Build history of the part. All positions in model axes, mm. A direction names the side the tool comes from. Give positions to 0.01 mm unless a question says otherwise; leave off trailing zeros. Loops run counter-clockwise (first coordinate to the right, second up) from the corner with the lowest first, then second, coordinate; pieces in that order, holes last.
1) Wall check: line 1 (X direction, y = -24.5, z = 0); line 2 (Z direction, x = 1, y = 50); line 3 (Z direction, x = -3.5, y = -19.5). Give the ranges that are in metal, low to high.
2) Band-saw the part on C-C on y = -2.5. List the corners of the cut face in (x, z).
3) Band-saw the part on A-A on y = -21.5. List the corners of the cut face in (x, z), then the cut area to 3 significant figures.
4) Flat gauge pins, fed straight in: P1, Ø8, axis at y = -17.5, z = 12, coming from the +X side; P2, Ø1, axis at x = -7, y = 41, coming from the +Z side; P3, Ø5, axis at x = 5.5, z = 0, coming from the -Y side. Where does each tip first touch, or does it go through?
5) Two-plate mould, pull along Z, no slides. Class faces 5 (the flat face through (-12.644, -18.94, 21.762)), 6 (the flat face through (30, 30, -1)), 7 (the flat face through (27.465, 0.103, -1.479)): +Z half, -Z half, draft (parallel to the pull), parting line (faces both ways), or undercut.
6) 3-axis set-ups, long thin cutter, end or side, ignore diameter. For faces 1 (the flat face through (0, -18, 10)), 2 (the flat face through (-21.755, -26.925, 10.331)), 3 (the flat face through (12.675, 0.103, -1.479)), 4 (the flat face through (2, 30, 0)): which of +Z, -Z, +X, -X, +Y, -Y reach the whole face in a straight line?
Autodesk Inventor part; units mm, degrees
ref_plane "YZ Plane" through (0, 0, 0) normal (1, 0, 0) x (0, 1, 0)
ref_plane "XZ Plane" through (0, 0, 0) normal (0, 1, 0) x (-1, 0, 0)
ref_plane "XY Plane" through (0, 0, 0) normal (0, 0, 1) x (1, 0, 0)
sketch "Skizze1" plane through (0, 0, 0) normal (1, 0, 0) x (0, 1, 0)
  line L0 (60, -3) -> (60, 0)
  line L1 (60, 0) -> (0, 0)
  line L2 (0, 0) -> (-10.8137, 24.3352)
  line L3 (-29, -3) -> (-30.8137, 22.9367)
  line L4 (-30.8137, 22.9367) -> (-10.8137, 24.3352)
  line L5 (-29, -3) -> (60, -3)
  dimension "d52" = 3
  dimension "d56" = 26
  dimension "d57" = 20
  dimension "d88" = 60
  dimension "d89" = 94
  dimension "d90" = 29
extrude "Extrusion1" add sketch "Skizze1" along normal mid plane 50
sketch "Skizze10" plane through (-25, -30.8137, 22.9367) normal (0, -0.0698, 0.9976) x (1, 0, 0)
  line L0 (50, 29.1386) -> (0, 29.1386)
  line L1 (25, 29.1386) -> (25, 0) construction
  line L2 (0, 0) -> (50, 0)
  line L3 (25, 0) -> (50, 0)
  line L4 (50, 0) -> (50, 29.1386)
  line L5 (50, 29.1386) -> (25, 29.1386)
  line L6 (25, 29.1386) -> (25, 0)
extrude "Extrusion8" cut sketch "Skizze10" against normal through all
sketch "Skizze17" plane through (-25, -30.8137, 22.9367) normal (0, -0.9976, -0.0698) x (1, 0, 0)
  circle A0 centre (12.5, -13) radius 7
  line L0 (25, -26) -> (25, 0)
  line L1 (25, 0) -> (0, 0)
  point P0 (25, -25.0302)
  point P1 (25, -13)
  point P2 (12.5, 0)
  dimension "d91" = 14
extrude "Extrusion13" cut sketch "Skizze17" against normal blind 3
sketch "Skizze18" plane through (-12.5, -26.9141, 10.1776) normal (0, -0.9976, -0.0698) x (1, 0, 0)
  line L0 (10.25, -11) -> (-10.25, -11)
  line L1 (-10.25, -11) -> (-10.25, 11)
  line L2 (-10.25, 11) -> (10.25, 11)
  line L3 (10.25, 11) -> (10.25, -11)
  line L4 (10.25, -11) -> (-10.25, 11) construction
  line L5 (-10.25, -11) -> (10.25, 11) construction
  line L6 (12.5, -13) -> (12.5, 13)
  line L7 (12.5, 13) -> (-12.5, 13)
  point P0 (12.5, -12.0302)
  point P1 (0, 0)
  point P2 (0, 0)
  point P3 (12.5, 0)
  point P4 (0, 0)
  point P5 (0, 13)
  dimension "d94" = 20.5
  dimension "d95" = 22
extrude "Extrusion14" cut sketch "Skizze18" against normal up to next
fillet "Rundung18" radius 2 1 edges at (-19.5, -26.9141, 10.1776)
fillet "Rundung19" radius 2 1 edges at (-12.5, -30.8137, 22.9367)
sketch "Skizze19" plane through (25, 0, 0) normal (1, 0, 0) x (0, 0, -1)
  line L0 (0, 0) -> (3, 0.2098)
  line L1 (3, 0.2098) -> (3, 60)
  line L2 (3, 60) -> (0, 60)
  line L3 (0, 60) -> (0, 0)
extrude "Extrusion15" add sketch "Skizze19" along normal blind 5
equation "\"G_L\" = 0"
equation "\"G_H\" = 0"
equation "\"G_B\" = 0"
properties part number "Airunit_aufnahme" material "GEDA Polyamid"
Findings below:
1. line 1: x = -25 to -22.75, -2.25 to 0
1. line 2: z = -3 to 0
1. line 3: z = -3 to -0.33, 21.72 to 23.73
2. outline: (-25, -3) - (0, -3) - (0, 5.63) - (-2.25, 5.63) - (-2.25, 0.86) - (-22.75, 0.86) - (-22.75, 5.63) - (-25, 5.63) - close
3. outline: (-25, -3) - (0, -3) - (0, 23.59) - (-25, 23.59) - close; hole (-22.75, -0.47) - (-2.25, -0.47) - (-2.25, 21.58) - (-22.75, 21.58) - close
3. area: 213 mm2
4. P1: stops at x = 0
4. P2: stops at z = 0
4. P3: stops at y = 0
5. face 5: undercut
5. face 6: draft
5. face 7: -Z half
6. face 1: +Z, -Z, +X, -Y
6. face 2: none
6. face 3: -Z, +X, -Y
6. face 4: +Z, +X, -X, +Y
